Verification items for the finished model (mm, model axes). A direction names the side the tool comes from. Give positions to 0.01 mm unless a question says otherwise; leave off trailing zeros. Loops run counter-clockwise (first coordinate to the right, second up) from the corner with the lowest first, then second, coordinate; pieces in that order, holes last. Notation, with made-up numbers: (39.25, 13.25) - (58.25, 13.25) arc R24 ccw to (58.25, 35.25) - close; hole circle Ø10 at (-30.5, 31). An arc over 180 degrees is marked (long way). Answer in a Markdown table with one row per item.
```python
from build123d import *

# Parameters (mm, degrees)
PAD_DEPTH       = 4
POCKET_DEPTH    = 4.5
SKETCH003_R     = 2.15
POCKET001_DEPTH = 7.001


with BuildPart() as part:
    # Sketch → Revolution (revolve)
    with BuildSketch(Plane.XZ):
        Polygon((0, 0), (9.344189, 0), (12, -4.6), (12, -7), (0, -7), align=None)
    revolve(axis=Axis((0, 0, 0), (0, 0, 1)))

    # Sketch002 → Pad (new body)
    with BuildSketch(Plane.YZ.offset(3.8)):
        with BuildLine():
            ThreePointArc((5, 6), (0, 11), (-5, 6))
            Line((-5, 6), (-5, 0))
            Line((-5, 0), (5, 0))
            Line((5, 6), (5, 0))
        make_face()
        with BuildLine():
            Line((-1.52028, 7.52028), (-0.890559, 8.15))
            Line((-0.890559, 8.15), (0.890559, 8.15))
            Line((0.890559, 8.15), (1.52028, 7.52028))
            ThreePointArc((-1.52028, 7.52028), (0, 3.85), (1.52028, 7.52028))
        make_face(mode=Mode.SUBTRACT)
    extrude(amount=PAD_DEPTH)

    # Sketch001 → Pocket (cut)
    with BuildSketch(Plane.XY):
        Polygon((3.6, 2.078461), (0, 4.156922), (-3.6, 2.078461), (-3.6, -2.078461), (0, -4.156922), (3.6, -2.078461), align=None)
    extrude(amount=-POCKET_DEPTH, mode=Mode.SUBTRACT)

    # Sketch003 → Pocket001 (cut, through all)
    with BuildSketch(Plane.XY):
        Circle(SKETCH003_R)
    extrude(amount=-POCKET001_DEPTH, mode=Mode.SUBTRACT)


solid = part.part
```
Q1. Go/stop test with flat-tipped pins: P1, Ø8, axis at y = -8.5, z = 2.5, coming from the +X side; P2, Ø1.2, axis at x = 6.5, z = 2, coming from the -Y side; P3, Ø6, axis at x = -7, y = 1, coming from the +Z side. Record where each tip stops, or that it passes through.
Completed:
| item | result |
|---|---|
| P1 | x = 7.8 |
| P2 | y = -5 |
| P3 | z = 0 |
Q2. Draft check along Y on faces 1 (the face through (3.8, 0, 3)), 2 (the face through (-2, -3, -2)), 3 (the face through (6, 0, 11)). Enter one of: +Y half, -Y half, draft (parallel to the pull), parting line (faces both ways), or undercut.
Completed:
| item | result |
|---|---|
| face 1 | draft |
| face 2 | undercut |
| face 3 | parting line |
Q3. Tool access check on faces 4 (the face through (-2, 3, -2)), 5 (the face through (6, 0, 8.15)), 6 (the face through (7.8, 0, 3)), 7 (the face through (-2.15, 0.09, -5.73)), 8 (the face through (6, -5, 3)). Record the directions out of +Z, -Z, +X, -X, +Y, -Y that give a thin tool (end or side, any length) a straight path to the whole face; none if there is none.
Completed:
| item | result |
|---|---|
| face 4 | +Z |
| face 5 | +X, -X |
| face 6 | +Z, +X, +Y, -Y |
| face 7 | +Z, -Z |
| face 8 | +Z, +X, -X, -Y |
Q4. Thickness scan on line 1 (Y direction, x = 6.35, z = 6); line 2 (Y direction, x = 0, z = -5.4); line 3 (Z direction, x = 4.9, y = 0). Record the ranges inside material, lowest first.
Completed:
| item | result |
|---|---|
| line 1 | -5 to -2.15, 2.15 to 5 |
| line 2 | -12 to -2.15, 2.15 to 12 |
| line 3 | -7 to 3.85, 8.15 to 11 |
Q5. Sectioned sample at B-B (z = 9.5). Record the cut outline in (x, y), and give its area (3 significant figures).
Completed:
| item | result |
|---|---|
| outline | (3.8, -3.57) - (7.8, -3.57) - (7.8, 3.57) - (3.8, 3.57) - close |
| area | 28.6 mm^2 |
Q6. Sectioned sample at A-A (y = 0). Record the cut outline in (x, z).
Completed:
| item | result |
|---|---|
| outline | (-12, -7) - (-2.15, -7) - (-2.15, -4.5) - (-3.6, -4.5) - (-3.6, 0) - (-9.34, 0) - (-12, -4.6) - close; (2.15, -7) - (12, -7) - (12, -4.6) - (9.34, 0) - (7.8, 0) - (7.8, 3.85) - (3.8, 3.85) - (3.8, 0) - (3.6, 0) - (3.6, -4.5) - (2.15, -4.5) - close; (3.8, 8.15) - (7.8, 8.15) - (7.8, 11) - (3.8, 11) - close |
